Check sheet for the modelled part. Datum: model origin and axes. Units: mm. A direction names the side the tool comes from. Coordinates: 2 decimals unless noted, no trailing zeros. Write each loop counter-clockwise with the first axis right and the second up, starting at its lowest first coordinate (ties: lowest second). Pieces come first, ordered by that corner, then holes. Notation, with made-up numbers: (16.5, -28.75) - (51.5, -28.75) arc R25 ccw to (51.5, -12.75) - close; hole circle Ø6 at (74.25, 51.25). An arc over 180 degrees is marked (long way). Write each question's results on one line, items separated by ' | '.
Autodesk Inventor part; units mm, degrees
ref_plane "YZ Plane" through (0, 0, 0) normal (1, 0, 0) x (0, 1, 0)
ref_plane "XZ Plane" through (0, 0, 0) normal (0, 1, 0) x (-1, 0, 0)
ref_plane "XY Plane" through (0, 0, 0) normal (0, 0, 1) x (1, 0, 0)
sketch "Boceto1" plane through (0, 0, 0) normal (0, 1, 0) x (-1, 0, 0)
  line L0 (-100, 75) -> (100, 75)
  line L1 (100, 75) -> (100, -75)
  line L2 (100, -75) -> (-100, -75)
  line L3 (-100, -75) -> (-100, 75)
  line L4 (-100, 75) -> (100, -75) construction
  line L5 (100, 75) -> (-100, -75) construction
  point P0 (0, 0)
  dimension "d0" = 200
  dimension "d1" = 150
extrude "Extrusión1" add sketch "Boceto1" along normal blind 3
sketch "Boceto2" plane through (0, 0, 0) normal (0, 1, 0) x (-1, 0, 0)
  line L0 (-100, -75) -> (100, -75)
  line L1 (100, -75) -> (100, 75)
  line L2 (100, 75) -> (-100, 75)
  line L3 (-100, 75) -> (-100, -75)
  line L4 (103, 78) -> (103, -78)
  line L5 (103, -78) -> (-103, -78)
  line L6 (-103, -78) -> (-103, 78)
  line L7 (-103, 78) -> (103, 78)
  point P0 (0, 0)
  dimension "d4" = 3
extrude "Extrusión2" add sketch "Boceto2" along normal blind 50
sketch "Boceto3" plane through (-103, 0, -78) normal (-1, 0, 0) x (0, 0, 1)
  line L0 (78, 0) -> (78, 50) construction
  line L1 (3, 50) -> (153, 50) construction
  line L2 (156, 0) -> (156, 50) construction
  line L3 (156, 25) -> (0.5528, 25) construction
  circle A0 centre (78.2764, 25) radius 3
  line L4 (0, 0) -> (156, 0)
  line L5 (156, 0) -> (156, 50)
  line L6 (0, 50) -> (156, 50)
  line L7 (0, 0) -> (0, 50)
  line L8 (0, 0) -> (156, 0)
  dimension "d7" = 6
  dimension "d11" = 25
extrude "Extrusión3" cut sketch "Boceto3" against normal blind 3 contours A0
sketch "Boceto4" plane through (-103, 0, 78) normal (0, 0, 1) x (1, 0, 0)
  line L0 (0, 0) -> (206, 0)
  line L1 (0, 25) -> (206, 25)
  circle A0 centre (92, 25) radius 9
  circle A1 centre (117, 25) radius 9
  line L2 (133, 18.25) -> (164, 18.25)
  line L3 (164, 18.25) -> (164, 31.75)
  line L4 (164, 31.75) -> (133, 31.75)
  line L5 (133, 31.75) -> (133, 18.25)
  line L6 (133, 18.25) -> (164, 31.75) construction
  line L7 (164, 18.25) -> (133, 31.75) construction
  line L8 (206, 0) -> (206, 50)
  line L9 (141.1134, 17.0625) -> (155.7384, 17.0625) construction
  line L10 (155.7384, 17.0625) -> (155.7384, 13.8861) construction
  line L11 (155.7384, 13.8861) -> (141.1134, 13.8861) construction
  line L12 (141.1134, 13.8861) -> (141.1134, 17.0625) construction
  spline S0 degree 2 poles (143.5785, 16.6501) (143.7514, 16.4475) (143.944, 15.8547) (143.944, 15.4743) knots 0 0 0 1 2 2 2
  spline S1 degree 2 poles (143.944, 15.4743) (143.944, 15.1038) (143.7563, 14.5036) (143.5785, 14.3011) knots 0 0 0 1 2 2 2
  spline S2 degree 2 poles (143.5785, 14.3011) (143.3907, 14.0886) (142.8943, 13.8861) (142.5954, 13.8861) knots 0 0 0 1 2 2 2
  spline S3 degree 2 poles (142.5954, 13.8861) (142.2866, 13.8861) (141.7926, 14.0961) (141.6123, 14.3011) knots 0 0 0 1 2 2 2
  spline S4 degree 2 poles (141.6123, 14.3011) (141.437, 14.5036) (141.2492, 15.0989) (141.2492, 15.4743) knots 0 0 0 1 2 2 2
  spline S5 degree 2 poles (141.2492, 15.4743) (141.2492, 15.8572) (141.4394, 16.4401) (141.6148, 16.6501) knots 0 0 0 1 2 2 2
  spline S6 degree 2 poles (141.6148, 16.6501) (141.7926, 16.8526) (142.2891, 17.0625) (142.5954, 17.0625) knots 0 0 0 1 2 2 2
  spline S7 degree 2 poles (142.5954, 17.0625) (142.9066, 17.0625) (143.4056, 16.8452) (143.5785, 16.6501) knots 0 0 0 1 2 2 2
  spline S8 degree 2 poles (143.5217, 15.4743) (143.5217, 15.7757) (143.3907, 16.2425) (143.2722, 16.3956) knots 0 0 0 1 2 2 2
  spline S9 degree 2 poles (143.2722, 16.3956) (143.1511, 16.5537) (142.8103, 16.7118) (142.5979, 16.7118) knots 0 0 0 1 2 2 2
  spline S10 degree 2 poles (142.5979, 16.7118) (142.378, 16.7118) (142.0471, 16.5587) (141.9211, 16.3956) knots 0 0 0 1 2 2 2
  spline S11 degree 2 poles (141.9211, 16.3956) (141.8, 16.24) (141.6716, 15.7707) (141.6716, 15.4743) knots 0 0 0 1 2 2 2
  spline S12 degree 2 poles (141.6716, 15.4743) (141.6716, 14.8741) (142.1755, 14.2368) (142.5979, 14.2368) knots 0 0 0 1 2 2 2
  spline S13 degree 2 poles (142.5979, 14.2368) (143.0202, 14.2368) (143.5217, 14.8741) (143.5217, 15.4743) knots 0 0 0 1 2 2 2
  line L13 (146.5697, 13.9503) -> (146.1152, 13.9503)
  line L14 (146.1152, 13.9503) -> (144.7665, 16.5784)
  line L15 (144.7665, 16.5784) -> (144.7665, 13.9503)
  line L16 (144.7665, 13.9503) -> (144.3886, 13.9503)
  line L17 (144.3886, 13.9503) -> (144.3886, 16.9983)
  line L18 (144.3886, 16.9983) -> (144.9641, 16.9983)
  line L19 (144.9641, 16.9983) -> (146.1917, 14.5851)
  line L20 (146.1917, 14.5851) -> (146.1917, 16.9983)
  line L21 (146.1917, 16.9983) -> (146.5697, 16.9983)
  line L22 (146.5697, 16.9983) -> (146.5697, 13.9503)
  line L23 (148.2172, 15.0989) -> (147.0637, 15.0989)
  line L24 (147.0637, 15.0989) -> (147.0637, 15.4694)
  line L25 (147.0637, 15.4694) -> (148.2172, 15.4694)
  line L26 (148.2172, 15.4694) -> (148.2172, 15.0989)
  spline S14 degree 2 poles (150.865, 16.6501) (151.0379, 16.4475) (151.2306, 15.8547) (151.2306, 15.4743) knots 0 0 0 1 2 2 2
  spline S15 degree 2 poles (151.2306, 15.4743) (151.2306, 15.1038) (151.0428, 14.5036) (150.865, 14.3011) knots 0 0 0 1 2 2 2
  spline S16 degree 2 poles (150.865, 14.3011) (150.6773, 14.0886) (150.1808, 13.8861) (149.8819, 13.8861) knots 0 0 0 1 2 2 2
  spline S17 degree 2 poles (149.8819, 13.8861) (149.5732, 13.8861) (149.0792, 14.0961) (148.8989, 14.3011) knots 0 0 0 1 2 2 2
  spline S18 degree 2 poles (148.8989, 14.3011) (148.7235, 14.5036) (148.5358, 15.0989) (148.5358, 15.4743) knots 0 0 0 1 2 2 2
  spline S19 degree 2 poles (148.5358, 15.4743) (148.5358, 15.8572) (148.726, 16.4401) (148.9013, 16.6501) knots 0 0 0 1 2 2 2
  spline S20 degree 2 poles (148.9013, 16.6501) (149.0792, 16.8526) (149.5757, 17.0625) (149.8819, 17.0625) knots 0 0 0 1 2 2 2
  spline S21 degree 2 poles (149.8819, 17.0625) (150.1932, 17.0625) (150.6921, 16.8452) (150.865, 16.6501) knots 0 0 0 1 2 2 2
  spline S22 degree 2 poles (150.8082, 15.4743) (150.8082, 15.7757) (150.6773, 16.2425) (150.5587, 16.3956) knots 0 0 0 1 2 2 2
  spline S23 degree 2 poles (150.5587, 16.3956) (150.4377, 16.5537) (150.0968, 16.7118) (149.8844, 16.7118) knots 0 0 0 1 2 2 2
  spline S24 degree 2 poles (149.8844, 16.7118) (149.6646, 16.7118) (149.3336, 16.5587) (149.2076, 16.3956) knots 0 0 0 1 2 2 2
  spline S25 degree 2 poles (149.2076, 16.3956) (149.0866, 16.24) (148.9582, 15.7707) (148.9582, 15.4743) knots 0 0 0 1 2 2 2
  spline S26 degree 2 poles (148.9582, 15.4743) (148.9582, 14.8741) (149.462, 14.2368) (149.8844, 14.2368) knots 0 0 0 1 2 2 2
  spline S27 degree 2 poles (149.8844, 14.2368) (150.3068, 14.2368) (150.8082, 14.8741) (150.8082, 15.4743) knots 0 0 0 1 2 2 2
  line L27 (153.498, 16.6377) -> (152.0803, 16.6377)
  line L28 (152.0803, 16.6377) -> (152.0803, 15.7781)
  line L29 (152.0803, 15.7781) -> (153.4388, 15.7781)
  line L30 (153.4388, 15.7781) -> (153.4388, 15.4175)
  line L31 (153.4388, 15.4175) -> (152.0803, 15.4175)
  line L32 (152.0803, 15.4175) -> (152.0803, 13.9503)
  line L33 (152.0803, 13.9503) -> (151.6752, 13.9503)
  line L34 (151.6752, 13.9503) -> (151.6752, 16.9983)
  line L35 (151.6752, 16.9983) -> (153.498, 16.9983)
  line L36 (153.498, 16.9983) -> (153.498, 16.6377)
  line L37 (155.684, 16.6377) -> (154.2662, 16.6377)
  line L38 (154.2662, 16.6377) -> (154.2662, 15.7781)
  line L39 (154.2662, 15.7781) -> (155.6247, 15.7781)
  line L40 (155.6247, 15.7781) -> (155.6247, 15.4175)
  line L41 (155.6247, 15.4175) -> (154.2662, 15.4175)
  line L42 (154.2662, 15.4175) -> (154.2662, 13.9503)
  line L43 (154.2662, 13.9503) -> (153.8611, 13.9503)
  line L44 (153.8611, 13.9503) -> (153.8611, 16.9983)
  line L45 (153.8611, 16.9983) -> (155.684, 16.9983)
  line L46 (155.684, 16.9983) -> (155.684, 16.6377)
  point P0 (103, 0)
  point P1 (148.5, 25)
  dimension "d0" = 200
  dimension "d1" = 150
  dimension "d10" = 25
  dimension "d12" = 18
  dimension "d13" = 18
  dimension "d14" = 31
  dimension "d15" = 13.5
  dimension "d16" = 42
  dimension "d17" = 25
  dimension "d18" = 16
extrude "Extrusión4" cut sketch "Boceto4" against normal blind 25 contours A0 L1 | L5 L4 L3 L1 | L1 L3 L2 L5 | A1 L1 | L1 A1 | L1 A0
extrude "Extrusión5" cut sketch "Boceto4" against normal blind 2 contours S0 S1 S2 S3 S4 S5 S6 S7 | L13 L14 L15 L16 L17 L18 L19 L20 L21 L22 | L23 L24 L25 L26 | S14 S15 S16 S17 S18 S19 S20 S21 | L27 L28 L29 L30 L31 L32 L33 L34 L35 L36 | L37 L38 L39 L40 L41 L42 L43 L44 L45 L46
sketch "Boceto5" plane through (-100, 3, -75) normal (0, 0, 1) x (1, 0, 0)
  line L0 (200, 0) -> (0, 0)
  line L1 (200, 0) -> (200, 47)
  line L2 (0, 47) -> (200, 47)
  line L3 (0, 0) -> (0, 47)
  point P0 (100, -3)
extrude "Extrusión6" cut sketch "Boceto5" against normal blind 3
sketch "Boceto6" plane through (0, 3, 0) normal (0, 1, 0) x (1, 0, 0)
  line L0 (-100, 78) -> (100, 78)
  line L1 (-100, 73) -> (100, 73) construction
  circle A0 centre (-90, 73) radius 2
  line L2 (-100, -75) -> (-100, 78)
  circle A1 centre (-30, 73) radius 2
  circle A2 centre (30, 73) radius 2
  circle A3 centre (90, 73) radius 2
  point P0 (0, 0)
  dimension "d25" = 5
  dimension "d26" = 4
  dimension "d27" = 10
  dimension "d30" = 60
extrude "Extrusión7" cut sketch "Boceto6" against normal blind 3
sketch "Boceto7" plane through (103, 0, 78) normal (1, 0, 0) x (0, 0, -1)
  line L0 (-0.5059, 25) -> (155.9287, 25) construction
  line L1 (156, 50) -> (3, 50) construction
  line L2 (25, 50) -> (25, 0) construction
  line L3 (0, 0) -> (0, 50) construction
  circle A0 centre (25, 25) radius 13.6
  point P0 (78, 0)
  dimension "d37" = 25
  dimension "d38" = 27.2
extrude "Extrusión8" cut sketch "Boceto7" against normal blind 3
equation "\"d19\" = d17"
properties part number "Chasis"
1. Sectioned sample at D-D (z = -52). Record the cut outline in (x, y), then the cut area to 3 significant figures.
Values follow:
outline: (-103, 0) - (103, 0) - (103, 50) - (100, 50) - (100, 3) - (-100, 3) - (-100, 50) - (-103, 50) - close | area: 900 mm^2
2. Sectioned sample at C-C (y = 25). Record the cut outline in (x, z).
Values follow:
outline: (-103, -78) - (-100, -78) - (-100, -2.72) - (-103, -2.72) - close; (-103, 3.28) - (-100, 3.28) - (-100, 75) - (-20, 75) - (-20, 78) - (-103, 78) - close; (-2, 75) - (5, 75) - (5, 78) - (-2, 78) - close; (23, 75) - (30, 75) - (30, 78) - (23, 78) - close; (61, 75) - (100, 75) - (100, 66.6) - (103, 66.6) - (103, 78) - (61, 78) - close; (100, -78) - (103, -78) - (103, 39.4) - (100, 39.4) - close
3. Material ranges on L1, parallel to X at y = 25, z = 76.6; L2, parallel to X at y = 12, z = -61; L3, parallel to Z at x = 30, y = 2, recorded low to high. Write a range as [from, to].
Values follow:
L1: x = [-103, -20], [-2, 5], [23, 30], [61, 103] | L2: x = [-103, -100], [100, 103] | L3: z = [-78, -75], [-71, 78]
4. Access from +Z, -Z, +X, -X, +Y, -Y to the whole of each face (thin tool, end or side, straight path). Record for faces 4 (the cylindrical face through (-101.52, 22.07, -0.37)), 5 (the flat face through (0.5, 50, 75.5)), 6 (the flat face through (-100, 21, 0)), 7 (the cylindrical face through (101.521, 34.192, 63.024)).
Values follow:
face 4: -X | face 5: +Z, -Z, +X, -X, +Y | face 6: -Z, +Y | face 7: +X
5. Sectioned sample at A-A (x = -11). Record the cut outline in (y, z), then the cut area to 3 significant figures.
Values follow:
outline: (0, -78) - (3, -78) - (3, 75) - (16, 75) - (16, 78) - (0, 78) - close; (34, 75) - (50, 75) - (50, 78) - (34, 78) - close | area: 555 mm^2
6. Sectioned sample at B-B (z = 53). Record the cut outline in (x, y), then the cut area to 3 significant figures.
Values follow:
outline: (-103, 0) - (103, 0) - (103, 11.4) - (100, 11.4) - (100, 3) - (-100, 3) - (-100, 50) - (-103, 50) - close; (100, 38.6) - (103, 38.6) - (103, 50) - (100, 50) - close | area: 818 mm^2
7. Draft check along Z on faces 1 (the flat face through (-1, 26, 75)), 2 (the cylindrical face through (91.075, 1.521, -74.686)), 3 (the flat face through (103, 25, -1)). Enter one of: pulls with the +Z half, pulls with the -Z half, needs draft (parallel to the pull), parting line crosses it, or undercut.
Values follow:
face 1: pulls with the -Z half | face 2: undercut | face 3: needs draft
